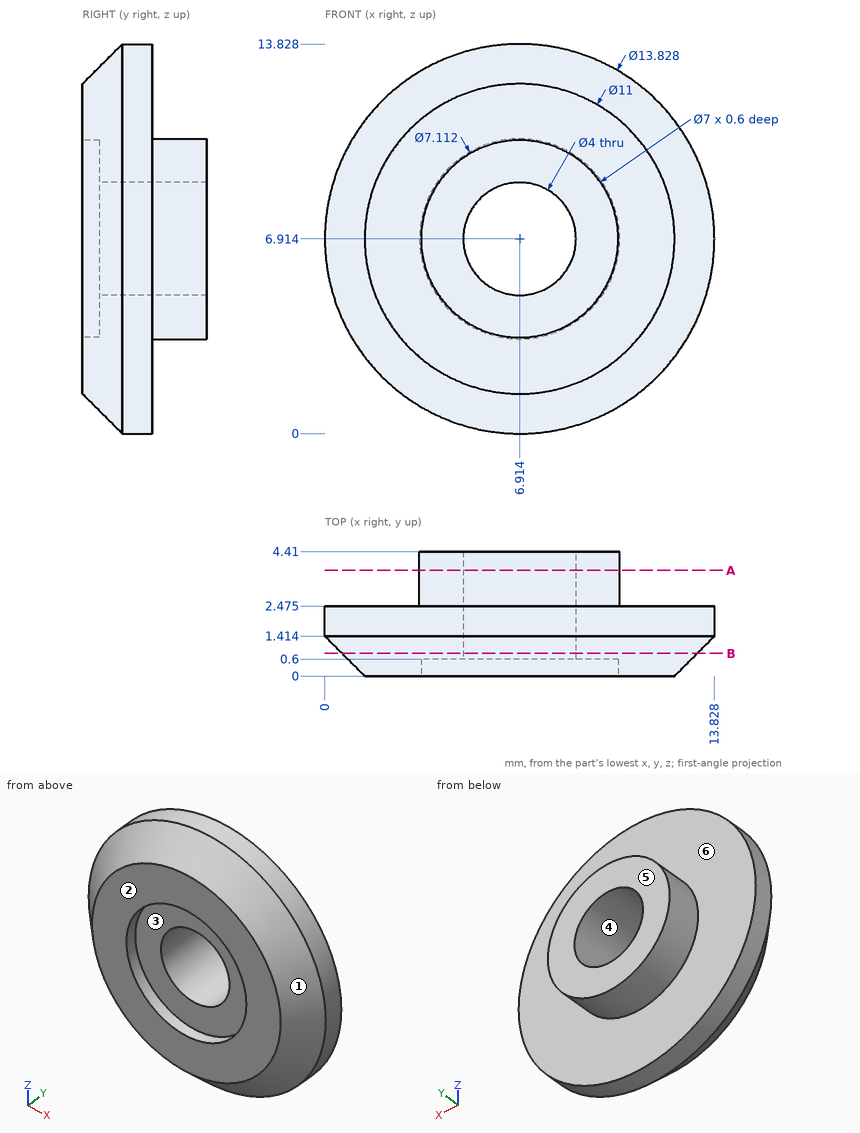
Can you work these out from the drawing? Everything is in mm from the part's minimum corner. A direction names the side the tool comes from. Give positions to 0.01 mm unless a question says otherwise; leave off trailing zeros. Write each loop counter-clockwise with the first axis right and the second up, starting at its lowest first coordinate (ties: lowest second). Pieces come first, ordered by that corner, then holes. Notation, with made-up numbers: (16.5, -24) -> (52.5, -24) arc R32 ccw to (52.5, 7) -> close; hole circle Ø7 at (-18, -16). An arc over 180 degrees is marked (long way). Write each question's results on one line, items separated by ' | '. Start each with the question number.
Q1. Which directions (+Z, -Z, +X, -X, +Y, -Y) give clear straight access to the entire face, cutting with the end or side of a thin tool? Please do the marked faces 5 and 6.
Q2. Suppose I cut it at A-A, the plane y = 3.75. List the corners of the cut face in (x, z) for me (1 decimal).
Q3. We'd pull the mould along X, two halves only. Please class the marked faces 1, 2, 3 and 4: +X half, -X half, draft (parallel to the pull), parting line (faces both ways), or undercut.
Q4. I need wall thicknesses on probe 1 along Z at (x, y) = (7, 2.9); probe 2 along X at (y, z) = (0.7, 8.5) (1 decimal). Which ranges of each line are inside material? Lowest first, please.
Q5. Suppose I cut it at B-B, the plane y = 0.8. List the corners of the cut face in (x, z) for me (1 decimal).
Q6. I'm going to push flat-ended pins straight in: pin 1 Ø1 at (x, y) = (9, 1.5) entering from -Z (1 decimal); pin 2 Ø2 at (x, z) = (6, 7.5) entering from -Y. Where does each tip first touch, or does it pass through?
Outcome:
1) face 5: +Z, -Z, +X, -X, +Y | face 6: +Y
2) outline: circle Ø7.1 at (6.9, 6.9); hole circle Ø4 at (6.9, 6.9)
3) face 1: parting line | face 2: draft | face 3: undercut | face 4: undercut
4) probe 1: 3.36 to 4.92, 8.91 to 10.47 | probe 2: 0.9 to 5.7, 8.1 to 12.9
5) outline: circle Ø12.6 at (6.9, 6.9); hole circle Ø4 at (6.9, 6.9)
6) pin 1: z = 0.2 | pin 2: y = 0.6
